Could you check a few things on this model? Use its own coordinates, in mm. Face numbers are marked on the shaded views. A direction names the side the tool comes from. Give positions to 0.01 mm unless a question says otherwise; leave off trailing zeros. Loops run counter-clockwise (first coordinate to the right, second up) from the corner with the lowest first, then second, coordinate; pieces in that order, holes last. Notation, with made-up numbers: M 11.5,29.25 L 25.5,29.25 A25 ccw 25.5,64.25 Z; hole C -34,85 d4. An arc over 180 degrees is marked long. Answer in a Markdown table with one row per item. Add a question column.
1. I'm going to push flat-ended pins straight in: pin 1 Ø4.5 at (x, y) = (-7, -5) entering from +Z; pin 2 Ø2 at (y, z) = (25, 5.5) entering from +X; pin 3 Ø4 at (x, z) = (-16, 12.5) entering from +Y. Where does each tip first touch, or does it pass through?
2. If we section it at B-B on z = 11: List the corners of the cut face in (x, y) for me, then the cut area to 3 significant figures.
3. If we section it at D-D on y = 10.5: List the corners of the cut face in (x, z) for me, then the cut area to 3 significant figures.
4. If we section it at C-C on z = -0.5: List the corners of the cut face in (x, y) for me.
5. Which directions (+Z, -Z, +X, -X, +Y, -Y) give clear straight access to the entire face, cutting with the end or side of a thin tool? Please do the marked faces 5, 6 and 7.
6. Thinking about a two-plate mould opening in Y: for the marked faces 1, 2, 3 and 4, which applies, released by +Y, released by -Y, zero draft, split by the parting line, or undercut?
7. I need wall thicknesses on line 1 along Y through (x, z) = (-7.5, -1.3); line 2 along X through (y, z) = (6.65, 7.5); line 3 along Y through (x, z) = (-12.5, 1.75). Which ranges of each line are inside material? Lowest first, please. Write a range as from..to.
8. If we section it at A-A on x = -13.9: List the corners of the cut face in (y, z) for me, then the cut area to 3 significant figures.
```python
from build123d import *

# Parameters (mm, degrees)
SKETCH1_W           = 40
SKETCH1_H           = 50
SKETCH1_R           = 1.25
BASE_FLANGE1_DEPTH  = 2.5
SKETCH15_R          = 1
CUT_EXTRUDE3_DEPTH  = 10
JOG3_START          = -2.5
JOG3_OUTLINE_W      = 40
JOG3_OUTLINE_H      = 48.294687966
JOG3_OUTLINE_R      = 1
JOG3_OUTLINE_R_2    = 1.25
JOG3_DEPTH          = 2.5
JOG3_2_OUTLINE_W    = 40
JOG3_2_OUTLINE_H    = 1.705312034
JOG3_2_DEPTH        = 0.332528284
JOG3_START_2        = 14.2634
JOG3_3_OUTLINE_W    = 40
JOG3_3_OUTLINE_H    = 35
JOG3_3_OUTLINE_R    = 1
JOG3_3_OUTLINE_R_2  = 1.25
JOG3_3_DEPTH        = 3.2366
JOG3_4_OUTLINE_W    = 40
JOG3_4_OUTLINE_H    = 15.794687966
JOG3_4_OUTLINE_R    = 1.25
JOG3_4_DEPTH        = 3.2366
JOG3_5_OUTLINE_W    = 40
JOG3_5_OUTLINE_H    = 2.5
JOG3_5_DEPTH        = 15
JOG3_START_3        = 15
JOG3_6_OUTLINE_R    = 1.25
JOG3_6_OUTLINE_R_2  = 1
JOG3_6_DEPTH        = 2.5
JOG3_START_4        = -20
JOG3_7_DEPTH        = 40
JOG4_START          = -20
JOG4_DEPTH          = 40
JOG4_2_DEPTH        = 40
JOG4_START_2        = -3
JOG4_3_OUTLINE_R    = 1.25
JOG4_3_DEPTH        = 4
FILLET1_R           = 10
SKETCH18_R          = 2.5
BOSS_EXTRUDE1_DEPTH = 2.5
SKETCH19_R          = 1
SKETCH19_W          = 23.5
SKETCH19_H          = 12.5
CUT_EXTRUDE4_DEPTH  = 2.5
SKETCH20_R          = 2.5
SKETCH20_R_2        = 1.25
CUT_EXTRUDE6_DEPTH  = 10
SKETCH23_R          = 2.5
CUT_EXTRUDE7_DEPTH  = 44.945989578
SKETCH24_R          = 5
CUT_EXTRUDE8_DEPTH  = 1.25
SKETCH25_W          = 20
SKETCH25_H          = 13.5268
CUT_EXTRUDE11_DEPTH = 50.640775238


with BuildPart() as part:
    # Base-Flange1: sheet metal written as solids
    # Sketch1 → Base-Flange1 (new body)
    with BuildSketch(Plane.XY):
        Rectangle(SKETCH1_W, SKETCH1_H)
        with Locations((10, 12.5)):
            Circle(SKETCH1_R, mode=Mode.SUBTRACT)
        with Locations(Location((10, -12.5, 0), (0, 0, 180))):
            Circle(SKETCH1_R, mode=Mode.SUBTRACT)
        with Locations((-10, -12.5)):
            Circle(SKETCH1_R, mode=Mode.SUBTRACT)
        with Locations(Location((-10, 12.5, 0), (0, 0, 180))):
            Circle(SKETCH1_R, mode=Mode.SUBTRACT)
    extrude(amount=-BASE_FLANGE1_DEPTH)

    # Sketch15 → Cut-Extrude3 (cut)
    with BuildSketch(Plane.XY):
        with Locations((12, 0)):
            Circle(SKETCH15_R)
        with Locations(Location((-17, 0, 0), (0, 0, 180))):
            Circle(SKETCH15_R)
    extrude(amount=-CUT_EXTRUDE3_DEPTH, mode=Mode.SUBTRACT)

    # Jog3: read off the stored shape, not the designer's step
    # Jog3 outline → Jog3 (cut)
    with BuildSketch(Plane.XY.offset(JOG3_START)):
        with Locations((0, -0.852656017)):
            Rectangle(JOG3_OUTLINE_W, JOG3_OUTLINE_H)
        with Locations((-17, 0)):
            Circle(JOG3_OUTLINE_R, mode=Mode.SUBTRACT)
        with Locations((12, 0)):
            Circle(JOG3_OUTLINE_R, mode=Mode.SUBTRACT)
        with Locations((-10, 12.5)):
            Circle(JOG3_OUTLINE_R_2, mode=Mode.SUBTRACT)
        with Locations((10, 12.5)):
            Circle(JOG3_OUTLINE_R_2, mode=Mode.SUBTRACT)
        with Locations((10, -12.5)):
            Circle(JOG3_OUTLINE_R_2, mode=Mode.SUBTRACT)
        with Locations((-10, -12.5)):
            Circle(JOG3_OUTLINE_R_2, mode=Mode.SUBTRACT)
    extrude(amount=JOG3_DEPTH, mode=Mode.SUBTRACT)

    # Jog3 2 outline → Jog3 2 (cut)
    with BuildSketch(Plane.XY.offset(JOG3_START)):
        with Locations((0, 24.147343983)):
            Rectangle(JOG3_2_OUTLINE_W, JOG3_2_OUTLINE_H)
    extrude(amount=JOG3_2_DEPTH, mode=Mode.SUBTRACT)

    # Jog3 4 outline → Jog3 4 (add)
    with BuildSketch(Plane.XY.offset(JOG3_START)):
        with Locations((0, 32.897343983)):
            Rectangle(JOG3_4_OUTLINE_W, JOG3_4_OUTLINE_H)
        with Locations((10, 28.294687966)):
            Circle(JOG3_4_OUTLINE_R, mode=Mode.SUBTRACT)
        with Locations((-10, 28.294687966)):
            Circle(JOG3_4_OUTLINE_R, mode=Mode.SUBTRACT)
    extrude(amount=JOG3_4_DEPTH)



with BuildPart() as body_2:
    # Jog3 3 outline → Jog3 3 (new body)
    with BuildSketch(Plane.XY.offset(JOG3_START_2)):
        with Locations((0, 8.294687966)):
            Rectangle(JOG3_3_OUTLINE_W, JOG3_3_OUTLINE_H)
        with Locations((12, 15.794687966)):
            Circle(JOG3_3_OUTLINE_R, mode=Mode.SUBTRACT)
        with Locations((-17, 0)):
            Circle(JOG3_3_OUTLINE_R, mode=Mode.SUBTRACT)
        with Locations((-10, 3.294687966)):
            Circle(JOG3_3_OUTLINE_R_2, mode=Mode.SUBTRACT)
        with Locations((12, 0)):
            Circle(JOG3_3_OUTLINE_R, mode=Mode.SUBTRACT)
        with Locations((10, 3.294687966)):
            Circle(JOG3_3_OUTLINE_R_2, mode=Mode.SUBTRACT)
        with Locations((-17, 15.794687966)):
            Circle(JOG3_3_OUTLINE_R, mode=Mode.SUBTRACT)
        with Locations((-10, 12.5)):
            Circle(JOG3_3_OUTLINE_R_2, mode=Mode.SUBTRACT)
        with Locations((10, 12.5)):
            Circle(JOG3_3_OUTLINE_R_2, mode=Mode.SUBTRACT)
    extrude(amount=JOG3_3_DEPTH)


with BuildPart() as part_1:
    add(part.part)

    add(body_2.part)  # Jog3 5 merges body 2
    # Jog3 5 outline → Jog3 5 (add)
    with BuildSketch(Plane.XY):
        with Locations((0, 24.544687966)):
            Rectangle(JOG3_5_OUTLINE_W, JOG3_5_OUTLINE_H)
    extrude(amount=JOG3_5_DEPTH)

    # Jog3 6 outline → Jog3 6 (add)
    with BuildSketch(Plane.XY.offset(JOG3_START_3)):
        with Locations((10, 12.5)):
            Circle(JOG3_6_OUTLINE_R)
        with Locations((-10, 12.5)):
            Circle(JOG3_6_OUTLINE_R)
        with Locations((12, 0)):
            Circle(JOG3_6_OUTLINE_R_2)
        with Locations((-17, 0)):
            Circle(JOG3_6_OUTLINE_R_2)
    extrude(amount=JOG3_6_DEPTH)

    # Jog3 7 outline → Jog3 7 (cut)
    with BuildSketch(Plane.YZ.offset(JOG3_START_4)):
        with BuildLine():
            ThreePointArc((23.294687966, 14.2634), (23.078942821, 14.784254855), (22.558087966, 15))
            Line((22.558087966, 15), (-9.205312034, 15))
            Line((-9.205312034, 15), (-9.205312034, 14.2634))
            Line((-9.205312034, 14.2634), (23.294687966, 14.2634))
        make_face()
        with BuildLine():
            ThreePointArc((26.531287966, -2.5), (24.242666158, -1.552021808), (23.294687966, 0.7366))
            Line((23.294687966, 0.7366), (23.294687966, -2.167471716))
            Line((23.294687966, -2.167471716), (25, -2.167471716))
            Line((25, -2.167471716), (25, -2.5))
            Line((25, -2.5), (26.531287966, -2.5))
        make_face()
        with BuildLine():
            Line((26.531287966, 0), (40.794687966, 0))
            Line((40.794687966, 0), (40.794687966, 0.7366))
            Line((40.794687966, 0.7366), (25.794687966, 0.7366))
            ThreePointArc((25.794687966, 0.7366), (26.010433111, 0.215745145), (26.531287966, 0))
        make_face()
        with BuildLine():
            Line((25.794687966, 17.5), (22.558087966, 17.5))
            ThreePointArc((22.558087966, 17.5), (24.846709774, 16.552021808), (25.794687966, 14.2634))
            Line((25.794687966, 14.2634), (25.794687966, 17.5))
        make_face()
    extrude(amount=JOG3_7_DEPTH, mode=Mode.SUBTRACT)

    # Jog4: read off the stored shape, not the designer's step
    # Jog4 outline → Jog4 (cut)
    with BuildSketch(Plane.YZ.offset(JOG4_START)):
        with BuildLine():
            Line((-9.205312034, 15), (5.87962174, 15))
            ThreePointArc((5.87962174, 15), (7.019882984, 16.799110859), (9.031287966, 17.5))
            Line((9.031287966, 17.5), (-9.205312034, 17.5))
            Line((-9.205312034, 17.5), (-9.205312034, 15))
        make_face()
    extrude(amount=JOG4_DEPTH, mode=Mode.SUBTRACT)

    # Jog4 2 outline → Jog4 2 (add)
    with BuildSketch(Plane.YZ.offset(JOG4_START)):
        with BuildLine():
            Line((-9.205312034, 0), (-9.205312034, -2.5))
            Line((-9.205312034, -2.5), (5.058087966, -2.5))
            ThreePointArc((5.058087966, -2.5), (7.346709774, -1.552021808), (8.294687966, 0.7366))
            Line((8.294687966, 0.7366), (8.294687966, 14.2634))
            ThreePointArc((8.294687966, 14.2634), (8.510433111, 14.784254855), (9.031287966, 15))
            Line((9.031287966, 15), (5.87962174, 15))
            ThreePointArc((5.87962174, 15), (5.81599152, 14.634140241), (5.794687966, 14.2634))
            Line((5.794687966, 14.2634), (5.794687966, 0.7366))
            ThreePointArc((5.794687966, 0.7366), (5.578942821, 0.215745145), (5.058087966, 0))
            Line((5.058087966, 0), (-9.205312034, 0))
        make_face()
    extrude(amount=JOG4_2_DEPTH)

    # Jog4 3 outline → Jog4 3 (cut)
    with BuildSketch(Plane.XY.offset(JOG4_START_2)):
        with Locations((-10, 3.294687966)):
            Circle(JOG4_3_OUTLINE_R)
        with Locations((10, 3.294687966)):
            Circle(JOG4_3_OUTLINE_R)
    extrude(amount=JOG4_3_DEPTH, mode=Mode.SUBTRACT)

    # Fillet1
    fillet1_edges = [part_1.edges().sort_by_distance(p)[0] for p in [
        (20, -9.205312034, -1.25),
        (-20, -9.205312034, -1.25),
        (-20, 40.794687966, -1.25),
        (20, 40.794687966, -1.25),
    ]]
    fillet(fillet1_edges, radius=FILLET1_R)

    # Sketch18 → Boss-Extrude1 (add)
    with BuildSketch(Plane.XY.offset(17.5)):
        with Locations((12, 15.794687966)):
            Circle(SKETCH18_R)
        with Locations((-17, 15.794687966)):
            Circle(SKETCH18_R)
    extrude(amount=-BOSS_EXTRUDE1_DEPTH)

    # Sketch19 → Cut-Extrude4 (cut)
    with BuildSketch(Plane(origin=(0, 25.794687966, 0), x_dir=(1, 0, 0), z_dir=(0, 1, 0))):
        with Locations(Location((13.9, -7.5, 0), (0, 0, 270))):
            Circle(SKETCH19_R)
        with Locations(Location((-13.9, -7.5, 0), (0, 0, 90))):
            Circle(SKETCH19_R)
        with Locations((0, -7.5)):
            Rectangle(SKETCH19_W, SKETCH19_H)
    extrude(amount=-CUT_EXTRUDE4_DEPTH, mode=Mode.SUBTRACT)

    # Sketch20 → Cut-Extrude6 (cut)
    with BuildSketch(Plane.XY):
        with Locations((0, 33.294687966)):
            Circle(SKETCH20_R)
        with Locations(Location((0, -1.705312034, 0), (0, 0, 180))):
            Circle(SKETCH20_R)
        with Locations((7.5, -1.705312034)):
            Circle(SKETCH20_R_2)
        with Locations(Location((-7.5, -1.705312034, 0), (0, 0, 180))):
            Circle(SKETCH20_R_2)
        with Locations(Location((7.5, 33.294687966, 0), (0, 0, 180))):
            Circle(SKETCH20_R_2)
        with Locations((-7.5, 33.294687966)):
            Circle(SKETCH20_R_2)
    extrude(amount=-CUT_EXTRUDE6_DEPTH, mode=Mode.SUBTRACT)

    # Sketch23 → Cut-Extrude7 (cut, through all)
    with BuildSketch(Plane(origin=(0, 25.794687966, 0), x_dir=(1, 0, 0), z_dir=(0, 1, 0))):
        with Locations(Location((-5.55, -7.5, 0), (0, 0, 270))):
            Circle(SKETCH23_R)
    extrude(amount=-CUT_EXTRUDE7_DEPTH, mode=Mode.SUBTRACT)

    # Sketch24 → Cut-Extrude8 (cut)
    with BuildSketch(Plane(origin=(0, 8.294687966, 0), x_dir=(1, 0, 0), z_dir=(0, 1, 0))):
        with Locations(Location((-5.55, -7.5, 0), (0, 0, 270))):
            Circle(SKETCH24_R)
    extrude(amount=-CUT_EXTRUDE8_DEPTH, mode=Mode.SUBTRACT)

    # Sketch25 → Cut-Extrude11 (cut, through all)
    with BuildSketch(Plane.XY.offset(17.5)):
        Polygon((20, 40.794687966), (0, 40.794687966), (0, 38.294687966), (-5, 38.294687966), (-5, 28.294687966), (0, 28.294687966), (0, 22.558087966), (20, 22.558087966), align=None)
        with Locations((10, 15.794687966)):
            Rectangle(SKETCH25_W, SKETCH25_H)
        Polygon((20, -9.205312034), (20, 9.031287966), (0, 9.031287966), (0, 3.294687966), (5, 3.294687966), (5, -6.705312034), (0, -6.705312034), (0, -9.205312034), align=None)
    extrude(amount=-CUT_EXTRUDE11_DEPTH, mode=Mode.SUBTRACT)


solid = part_1.part
```
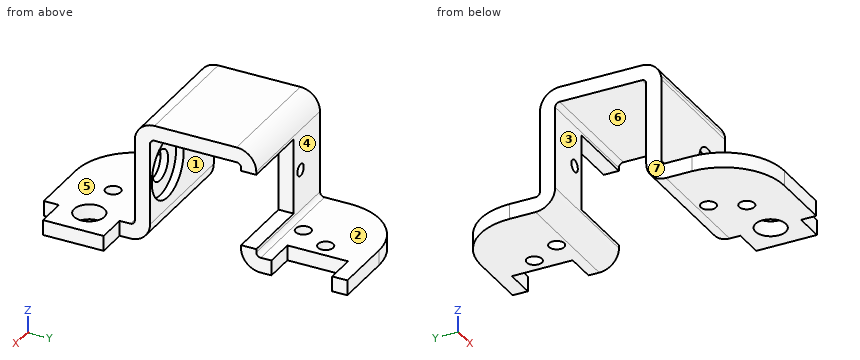
Results:
| question | item | result |
|---|---|---|
| 1 | pin 1 | z = 0 |
| 1 | pin 2 | x = -11.75 |
| 1 | pin 3 | y = 25.79 |
| 2 | outline | M -20,5.79 L 0,5.79 L 0,8.29 L -1.98,8.29 L -1.98,7.04 L -9.12,7.04 L -9.12,8.29 L -20,8.29 Z; M -20,23.29 L -11.75,23.29 L -11.75,25.79 L -20,25.79 Z |
| 2 | area | 61.7 mm2 |
| 3 | outline | M -20,15 L 0,15 L 0,17.5 L -20,17.5 Z |
| 3 | area | 50.0 mm2 |
| 4 | outline | M -20,0.79 A10 ccw -10,-9.21 L 0,-9.21 L 0,-6.71 L 5,-6.71 L 5,3.29 L 0,3.29 L 0,8.05 L -20,8.05 Z; M -20,23.54 L 0,23.54 L 0,28.29 L -5,28.29 L -5,38.29 L 0,38.29 L 0,40.79 L -10,40.79 A10 ccw -20,30.79 Z; hole C -10,3.29 d2.5; hole C -10,28.29 d2.5; hole C -7.5,-1.71 d2.5; hole C -7.5,33.29 d2.5; hole C 0,-1.71 d5 |
| 5 | face 5 | +Z, +X, -X, -Y |
| 5 | face 6 | -Z, +X, -X |
| 5 | face 7 | +Z, -Z, -X, +Y, -Y |
| 6 | face 1 | undercut |
| 6 | face 2 | zero draft |
| 6 | face 3 | undercut |
| 6 | face 4 | released by +Y |
| 7 | line 1 | -9.21..-2.96, -0.46..7.57, 24.02..32.04, 34.54..40.79 |
| 7 | line 2 | -20..-8.05, -3.05..0 |
| 7 | line 3 | 5.79..8.29, 23.29..25.79 |
| 8 | outline | M -8.41,-2.5 L 5.06,-2.5 A3.24 ccw 8.29,0.74 L 8.29,14.26 A0.74 cw 9.03,15 L 22.56,15 A0.74 cw 23.29,14.26 L 23.29,8.5 L 25.79,8.5 L 25.79,14.26 A3.24 ccw 22.56,17.5 L 9.03,17.5 A3.24 ccw 5.79,14.26 L 5.79,0.74 A0.74 cw 5.06,0 L -8.41,0 Z; M 23.29,0.74 A3.24 ccw 26.53,-2.5 L 40,-2.5 L 40,0 L 26.53,0 A0.74 cw 25.79,0.74 L 25.79,6.5 L 23.29,6.5 Z |
| 8 | area | 195 mm2 |
